from build123d import *

# Parameters (mm, degrees)
SKETCH1_W              = 20
SKETCH1_H              = 4
BOSS_EXTRUDE1_DEPTH    = 10
M8X1_25_TAPPED_HOLE1_D = 6.8


with BuildPart() as part:
    # Sketch1 → Boss-Extrude1 (new, symmetric)
    with BuildSketch(Plane.XY):
        Rectangle(SKETCH1_W, SKETCH1_H)
    extrude(amount=BOSS_EXTRUDE1_DEPTH, both=True)

    # M8x1.25 Tapped Hole1 (through all)
    with Locations(Plane(origin=(0, 2, 0), x_dir=(1, 0, 0), z_dir=(0, 1, 0))):
        with Locations((0, 0)):
            Hole(M8X1_25_TAPPED_HOLE1_D / 2)


solid = part.part
Can you work these out from the model? Positions are in its coordinate system, mm. Coordinates: 2 decimals unless noted, no trailing zeros. Loops run counter-clockwise (first coordinate to the right, second up) from the corner with the lowest first, then second, coordinate; pieces in that order, holes last. Notation, with made-up numbers: (-28.5, 35.5) - (-17.5, 35.5) arc R20 ccw to (-17.5, 50.5) - close; hole circle Ø10 at (39, 56.25). An arc over 180 degrees is marked (long way). Answer as a JSON object with one key per item and string values. Group by question number.
Item 1: If we section it at C-C (y = -0.8): List the corners of the cut face in (x, z) for me, plus the area to 3 significant figures.
Item 2: If I drill on L1, parallel to Z at x = 0, y = -0.5; L2, parallel to Z at x = -1.5, y = 1.5; L3, parallel to X at y = -0.25, z = 3, over which ranges is the centre line in solid material (lowest first)? Write a range as from..to.
Item 3: If we section it at A-A (z = 3): List the corners of the cut face in (x, y) for me.
Item 4: If we mould it in two halves opening along Z, with no side actions, what happens to faces 1 (the face through (0, 0, -10)), 2 (the face through (0, 0, 10)), 3 (the face through (-10, 0, 0)), 4 (the face through (0.74, -0.03, 3.32))? For each: released by +Z, released by -Z, zero draft, split by the parting line, or undercut.
Item 5: If we section it at B-B (x = 0): List the corners of the cut face in (y, z) for me.
Returned:
{
 "1": {"outline": "(-10, -10) - (10, -10) - (10, 10) - (-10, 10) - close; hole circle Ø6.8 at (0, 0)", "area": "364 mm²"},
 "2": {"L1": "z = -10..-3.4, 3.4..10", "L2": "z = -10..-3.05, 3.05..10", "L3": "x = -10..-1.6, 1.6..10"},
 "3": {"outline": "(-10, -2) - (-1.6, -2) - (-1.6, 2) - (-10, 2) - close; (1.6, -2) - (10, -2) - (10, 2) - (1.6, 2) - close"},
 "4": {"face 1": "released by -Z", "face 2": "released by +Z", "face 3": "zero draft", "face 4": "undercut"},
 "5": {"outline": "(-2, -10) - (2, -10) - (2, -3.4) - (-2, -3.4) - close; (-2, 3.4) - (2, 3.4) - (2, 10) - (-2, 10) - close"}
}
